Geometry check sheet. Reference: the model listing, model coordinates, mm. Face numbers are marked on the shaded views. A direction names the side the tool comes from. Round coordinates to 2 decimals unless told otherwise and drop trailing zeros. Order: outer loops, then holes, each group sorted by start corner. A loop starts at its lowest first (then second) coordinate and runs counter-clockwise, first axis right, second up. Notation, with made-up numbers: (-35.75, 8.25) - (12.25, 8.25) arc R22 cw to (12.25, 22.25) - close; hole circle Ø7 at (-3, 23). An arc over 180 degrees is marked (long way). Use a Markdown table: item, result. Add a question column.
(1) Thickness scan on line 1 along X through (y, z) = (25, 0); line 2 along X through (y, z) = (24.5, 1); line 3 along Y through (x, z) = (8.5, -1) (3 decimals). Record the ranges inside material, lowest first. Write a range as [from, to].
(2) Section check B-B on z = 0. Record the boundary of the cut face in (x, y) (1 decimal).
(3) Section check C-C on y = 29.5. Record the boundary of the cut face in (x, z).
(4) Access from +Z, -Z, +X, -X, +Y, -Y to the whole of each face (thin tool, end or side, straight path). Record for the marked faces 1, 2 and 3.
(5) Gauge pin test, flat ends, axial feed: P1, Ø3, axis at x = 9.5, z = -4.5, coming from the +Y side (3 decimals); P2, Ø1.5, axis at x = -4.5, y = 11, coming from the -Z side; P3, Ø4, axis at y = 18.5, z = 6.5, coming from the -X side. Record the tip position at first contact, or that the pin passes through.
(6) Section check A-A on x = 0. Record the boundary of the cut face in (y, z), then the cut area to 3 significant figures.
(7) Mould release check, pull along X, two halves, no side actions. Record for the marked faces 4, 5 and 6: released by +X, released by -X, zero draft, split by the parting line, or undercut.
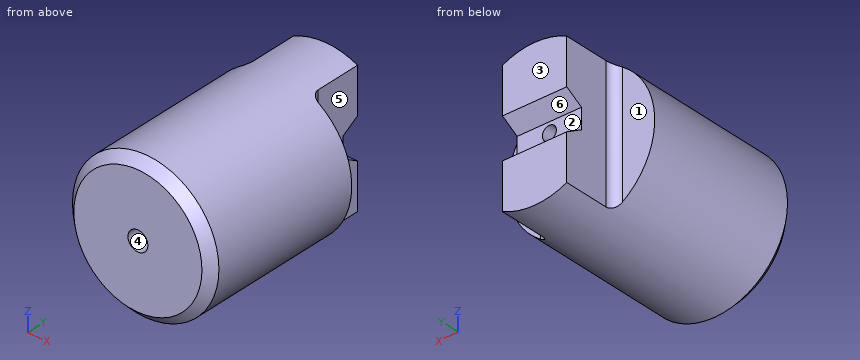
```python
from build123d import *

# Parameters (mm, degrees)
CROQUIS1_R                  = 12.6746
SALIENTE_EXTRUIR1_DEPTH     = 38.1
CORTAR_EXTRUIR1_DEPTH       = 43.105830598
CORTAR_EXTRUIR1_DEPTH_BACK  = 43.105830598
CORTAR_EXTRUIR2_DEPTH       = 43.105830598
CORTAR_EXTRUIR2_DEPTH_BACK  = 43.105830598
CHAFL_N1_SIZE               = 1.5875
CROQUIS4_R                  = 1.2192
CORTAR_EXTRUIR3_DEPTH       = 43.105830748
TALADRO_ROSCADO_8_321_D     = 3.4544
TALADRO_ROSCADO_8_321_DEPTH = 20.574
TALADRO_ROSCADO_8_321_TIP   = 1.037806461


with BuildPart() as part:
    # Croquis1 → Saliente-Extruir1 (new body)
    with BuildSketch(Plane(origin=(0, 0, 0), x_dir=(1, 0, 0), z_dir=(0, 1, 0))):
        with Locations(Location((0, 0, 0), (0, 0, 90))):
            Circle(CROQUIS1_R)
    extrude(amount=SALIENTE_EXTRUIR1_DEPTH)

    # Croquis2 → Cortar-Extruir1 (cut, two sides: drawn at the far end of the back side and taken through both)
    with BuildSketch(Plane(origin=(0, 0, 0), x_dir=(0, 0, -1), z_dir=(1, 0, 0)).offset(-CORTAR_EXTRUIR1_DEPTH_BACK)):
        Polygon((-3.5052, 38.1), (3.5052, 38.1), (1.7526, 35.1028), (-1.7526, 35.1028), align=None)
    extrude(amount=CORTAR_EXTRUIR1_DEPTH + CORTAR_EXTRUIR1_DEPTH_BACK, mode=Mode.SUBTRACT)

    # Croquis3 → Cortar-Extruir2 (cut, two sides: drawn at the far end of the back side and taken through both)
    with BuildSketch(Plane.XY.offset(-CORTAR_EXTRUIR2_DEPTH_BACK)):
        with BuildLine():
            Line((-12.6746, 28.575), (-7.0866, 28.575))
            ThreePointArc((-7.0866, 28.575), (-6.008969265, 29.021369265), (-5.5626, 30.099))
            Line((-5.5626, 30.099), (-5.5626, 38.1))
            Line((-5.5626, 38.1), (-12.6746, 38.1))
            Line((-12.6746, 38.1), (-12.6746, 28.575))
        make_face()
        with BuildLine():
            Line((12.6746, 38.1), (12.6746, 28.575))
            Line((12.6746, 28.575), (7.0866, 28.575))
            ThreePointArc((7.0866, 28.575), (6.008969265, 29.021369265), (5.5626, 30.099))
            Line((5.5626, 30.099), (5.5626, 38.1))
            Line((5.5626, 38.1), (12.6746, 38.1))
        make_face()
    extrude(amount=CORTAR_EXTRUIR2_DEPTH + CORTAR_EXTRUIR2_DEPTH_BACK, mode=Mode.SUBTRACT)

    # Chaflán1
    chafl_n1_edges = [part.edges().sort_by_distance(p)[0] for p in [
        (0, 0, 12.6746),
    ]]
    chamfer(chafl_n1_edges, length=CHAFL_N1_SIZE)

    # Croquis4 → Cortar-Extruir3 (cut, through all)
    with BuildSketch(Plane.XZ):
        with Locations(Location((0, 0, 0), (0, 0, 270))):
            Circle(CROQUIS4_R)
    extrude(amount=-CORTAR_EXTRUIR3_DEPTH, mode=Mode.SUBTRACT)

    # Taladro roscado #8-321
    with Locations(Plane(origin=(0, 0, 0), x_dir=(-1, 0, 0), z_dir=(0, -1, 0))):
        with Locations((0, 0)):
            Hole(TALADRO_ROSCADO_8_321_D / 2, depth=TALADRO_ROSCADO_8_321_DEPTH)
            with Locations((0, 0, -(TALADRO_ROSCADO_8_321_DEPTH + TALADRO_ROSCADO_8_321_TIP / 2))):  # 118° drill point
                Cone(0, TALADRO_ROSCADO_8_321_D / 2, TALADRO_ROSCADO_8_321_TIP, mode=Mode.SUBTRACT)


solid = part.part
```
Check sheet entries:
| question | item | result |
|---|---|---|
| 1 | line 1 | x = [-12.67, -1.22], [1.22, 12.67] |
| 1 | line 2 | x = [-12.64, -0.7], [0.7, 12.64] |
| 1 | line 3 | y = [0, 28.575] |
| 2 | outline | (-12.7, 1.6) - (-11.1, 0) - (-1.7, 0) - (-1.7, 20.6) - (-1.2, 20.9) - (-1.2, 35.1) - (-5.6, 35.1) - (-5.6, 30.1) arc R1.5 cw to (-7.1, 28.6) - (-12.7, 28.6) - close; (1.2, 20.9) - (1.7, 20.6) - (1.7, 0) - (11.1, 0) - (12.7, 1.6) - (12.7, 28.6) - (7.1, 28.6) arc R1.5 cw to (5.6, 30.1) - (5.6, 35.1) - (1.2, 35.1) - close |
| 3 | outline | (-5.69, -11.33) arc R12.67 ccw to (5.69, -11.33) - (5.69, 11.33) arc R12.67 ccw to (-5.69, 11.33) - close; hole circle Ø2.44 at (0, 0) |
| 4 | face 1 | +Z, -Z, -X, +Y |
| 4 | face 2 | +X, -X, +Y |
| 4 | face 3 | +Z, -Z, +X, -X, +Y |
| 5 | P1 | stops at y = 28.575 |
| 5 | P2 | stops at z = -12.11 |
| 5 | P3 | stops at x = -11.85 |
| 6 | outline | (0, -11.09) - (1.59, -12.67) - (38.1, -12.67) - (38.1, -3.51) - (35.1, -1.75) - (35.1, -1.22) - (20.88, -1.22) - (20.57, -1.73) - (0, -1.73) - close; (0, 1.73) - (20.57, 1.73) - (20.88, 1.22) - (35.1, 1.22) - (35.1, 1.75) - (38.1, 3.51) - (38.1, 12.67) - (1.59, 12.67) - (0, 11.09) - close |
| 6 | area | 841 mm2 |
| 7 | face 4 | undercut |
| 7 | face 5 | released by +X |
| 7 | face 6 | zero draft |
